from build123d import *

# Parameters (mm, degrees)
SKETCH1_R           = 3.7592
SKETCH1_R_2         = 0.6096
BOSS_EXTRUDE1_DEPTH = 1.5875
FILLET1_R           = 1.905
FILLET2_R           = 1.905


with BuildPart() as part:
    # Sketch1 → Boss-Extrude1 (new body)
    with BuildSketch(Plane.XY):
        with BuildLine():
            Line((34.29, -22.225), (33.367605666, -11.9888))
            ThreePointArc((33.367605666, -11.9888), (32.635899737, 4.284200971), (30.44668746, 20.425864572))
            ThreePointArc((30.44668746, 20.425864572), (27.794074787, 25.778474462), (22.225, 27.94))
            Line((22.225, 27.94), (-22.225, 27.94))
            ThreePointArc((-22.225, 27.94), (-27.794074787, 25.778474462), (-30.44668746, 20.425864572))
            ThreePointArc((-30.44668746, 20.425864572), (-32.635899737, 4.284200971), (-33.367605666, -11.9888))
            Line((-33.367605666, -11.9888), (-34.29, -22.225))
            Line((-34.29, -22.225), (-19.719346062, -22.225))
            ThreePointArc((-19.719346062, -22.225), (-19.755004666, -21.229024189), (-18.886028855, -21.717))
            ThreePointArc((-18.886028855, -21.717), (-18.969553044, -22.014475811), (-19.195711648, -22.225))
            Line((-19.195711648, -22.225), (19.195711648, -22.225))
            ThreePointArc((19.195711648, -22.225), (19.160053044, -21.229024189), (20.029028855, -21.717))
            ThreePointArc((20.029028855, -21.717), (19.945504666, -22.014475811), (19.719346062, -22.225))
            Line((19.719346062, -22.225), (34.29, -22.225))
        make_face()
        Polygon((-5.1562, -19.939), (-30.110080889, -19.939), (-30.110080889, -17.78), (-31.888080889, -17.78), (-31.888080889, -16.002), (-30.110080889, -16.002), (-30.110080889, -10.033), (-5.1562, -10.033), (-5.1562, -16.002), (-4.456080889, -16.002), (-4.456080889, -17.78), (-5.1562, -17.78), align=None, mode=Mode.SUBTRACT)
        with Locations((0, -15.748)):
            Circle(SKETCH1_R, mode=Mode.SUBTRACT)
        Polygon((5.1562, -19.939), (5.1562, -17.78), (4.456080889, -17.78), (4.456080889, -16.002), (5.1562, -16.002), (5.1562, -10.033), (30.110080889, -10.033), (30.110080889, -16.002), (31.888080889, -16.002), (31.888080889, -17.78), (30.110080889, -17.78), (30.110080889, -19.939), align=None, mode=Mode.SUBTRACT)
        with BuildLine():
            Line((-16.907947674, 25.654), (16.907947674, 25.654))
            ThreePointArc((16.907947674, 25.654), (17.978031977, 25.210756569), (18.421275408, 24.140672267))
            Line((18.421275408, 24.140672267), (18.421275408, 24.136275408))
            ThreePointArc((18.421275408, 24.136275408), (18.793249795, 23.238249795), (19.691275408, 22.866275408))
            Line((19.691275408, 22.866275408), (20.186724592, 22.866275408))
            ThreePointArc((20.186724592, 22.866275408), (21.084750205, 23.238249795), (21.456724592, 24.136275408))
            Line((21.456724592, 24.136275408), (21.456724592, 24.871259676))
            ThreePointArc((21.456724592, 24.871259676), (21.686749328, 25.425496663), (22.24162483, 25.653976848))
            ThreePointArc((22.24162483, 25.653976848), (26.292824304, 24.053268127), (28.177671702, 20.126203591))
            ThreePointArc((28.177671702, 20.126203591), (29.260117929, 13.484694907), (30.092217203, 6.8072))
            Line((30.092217203, 6.8072), (27.552217203, 6.8072))
            Line((27.552217203, 6.8072), (27.552217203, 4.9022))
            Line((27.552217203, 4.9022), (29.457217203, 4.9022))
            Line((29.457217203, 4.9022), (29.457217203, 3.175))
            Line((29.457217203, 3.175), (27.552217203, 3.175))
            Line((27.552217203, 3.175), (27.552217203, 1.27))
            Line((27.552217203, 1.27), (29.457217203, 1.27))
            Line((29.457217203, 1.27), (29.457217203, -5.0038))
            Line((29.457217203, -5.0038), (27.552217203, -5.0038))
            Line((27.552217203, -5.0038), (27.552217203, -6.2738))
            Line((27.552217203, -6.2738), (29.457217203, -6.2738))
            Line((29.457217203, -6.2738), (29.457217203, -8.001))
            Line((29.457217203, -8.001), (-29.457217203, -8.001))
            Line((-29.457217203, -8.001), (-29.457217203, -6.2738))
            Line((-29.457217203, -6.2738), (-27.552217203, -6.2738))
            Line((-27.552217203, -6.2738), (-27.552217203, -5.0038))
            Line((-27.552217203, -5.0038), (-29.457217203, -5.0038))
            Line((-29.457217203, -5.0038), (-29.457217203, 1.27))
            Line((-29.457217203, 1.27), (-27.552217203, 1.27))
            Line((-27.552217203, 1.27), (-27.552217203, 3.175))
            Line((-27.552217203, 3.175), (-29.457217203, 3.175))
            Line((-29.457217203, 3.175), (-29.457217203, 4.9022))
            Line((-29.457217203, 4.9022), (-27.552217203, 4.9022))
            Line((-27.552217203, 4.9022), (-27.552217203, 6.8072))
            Line((-27.552217203, 6.8072), (-30.092217203, 6.8072))
            ThreePointArc((-30.092217203, 6.8072), (-29.260117929, 13.484694907), (-28.177671702, 20.126203591))
            ThreePointArc((-28.177671702, 20.126203591), (-26.292824304, 24.053268127), (-22.24162483, 25.653976848))
            ThreePointArc((-22.24162483, 25.653976848), (-21.686749328, 25.425496663), (-21.456724592, 24.871259676))
            Line((-21.456724592, 24.871259676), (-21.456724592, 24.136275408))
            ThreePointArc((-21.456724592, 24.136275408), (-21.084750205, 23.238249795), (-20.186724592, 22.866275408))
            Line((-20.186724592, 22.866275408), (-19.691275408, 22.866275408))
            ThreePointArc((-19.691275408, 22.866275408), (-18.793249795, 23.238249795), (-18.421275408, 24.136275408))
            Line((-18.421275408, 24.136275408), (-18.421275408, 24.140672267))
            ThreePointArc((-18.421275408, 24.140672267), (-17.978031977, 25.210756569), (-16.907947674, 25.654))
        make_face(mode=Mode.SUBTRACT)
        with Locations((-19.939, 24.384)):
            Circle(SKETCH1_R_2, mode=Mode.SUBTRACT)
        with Locations((19.939, 24.384)):
            Circle(SKETCH1_R_2, mode=Mode.SUBTRACT)
    extrude(amount=BOSS_EXTRUDE1_DEPTH)

    # Fillet1
    fillet1_edges = [part.edges().sort_by_distance(p)[0] for p in [
        (5.1562, -19.939, 0.79375),
        (30.110080889, -19.939, 0.79375),
        (30.110080889, -10.033, 0.79375),
        (5.1562, -10.033, 0.79375),
        (-5.1562, -19.939, 0.79375),
        (-5.1562, -10.033, 0.79375),
        (-30.110080889, -10.033, 0.79375),
        (-30.110080889, -19.939, 0.79375),
    ]]
    fillet(fillet1_edges, radius=FILLET1_R)

    # Fillet2
    fillet2_edges = [part.edges().sort_by_distance(p)[0] for p in [
        (-29.457217203, 1.27, 0.79375),
        (-29.457217203, -5.0038, 0.79375),
        (-30.092217203, 6.8072, 0.79375),
        (29.457217203, -5.0038, 0.79375),
        (29.457217203, 1.27, 0.79375),
        (30.092217203, 6.8072, 0.79375),
    ]]
    fillet(fillet2_edges, radius=FILLET2_R - 0.0001)  # a hair under: the kernel refuses the full size


solid = part.part
Input: part model. Units: mm. Frame: model coordinates. A direction names the side the tool comes from. Coordinates: 2 decimals unless noted, no trailing zeros. Loops run counter-clockwise (first coordinate to the right, second up) from the corner with the lowest first, then second, coordinate; pieces in that order, holes last.
Q1. Contact query for flat-ended pins moving along their axis: pin 1 (0.5 mm diameter, centred on y = -17, z = 0.5, fed in from +X); pin 2 (2 mm diameter, centred on x = -19.939, y = 24.384, fed in from -Z); pin 3 (0.8 mm diameter, centred on y = 4.5, z = 0.5, fed in from -X); pin 4 (0.8 mm diameter, centred on y = -14.5, z = 1, fed in from +X). Output: stop coordinate, or through.
Q2. Draft query along X for faces 1 (the face through (29.57, -10.61, 0.8)), 2 (the face through (33.835, -17.179, 0.783)), 3 (the face through (-27.731, 25.836, 0.783)). Return one class per face: +X half, -X half, draft (parallel to the pull), parting line (faces both ways), or undercut.
Q3. Set-up query: faces 4 (the face through (5.156, -14, 1)), 5 (the face through (-0.2, -8.2, 1.588)). Return all of +Z, -Z, +X, -X, +Y, -Y with unobstructed straight access to the full face (end or side cutting, diameter ignored); none if empty.
Q4. Material intervals for line 1 (Y direction, x = -9, z = 0.6) (3 decimals); line 2 (Y direction, x = 0, z = 1.15) (3 decimals); line 3 (X direction, y = 24.5, z = 0.2), sorted ascending.
Q5. Cut plane D-D (z = 0.9). Give the number of separate pieces and of enclosed holes in the cut face, then the cut area to 3 significant figures.
Q6. Cut plane A-A (x = 13). Output: boundary loops of the cut face in (y, z) (1 decimal).
Q7. Cut plane C-C (x = 0). Output: boundary loops of the cut face in (y, z) (1 decimal), then the cut area to 3 significant figures.
Q8. Cut plane B-B (y = 13.5). Output: boundary loops of the cut face in (x, z).
Working result:
1. pin 1: stops at x = 33.84
1. pin 2: stops at z = 0
1. pin 3: stops at x = -32.65
1. pin 4: stops at x = 33.63
2. face 1: undercut
2. face 2: +X half
2. face 3: -X half
3. face 4: +Z, -Z
3. face 5: +Z, +X, -X, +Y, -Y
4. line 1: y = -22.225 to -19.939, -10.033 to -8.001, 25.654 to 27.94
4. line 2: y = -22.225 to -19.507, -11.989 to -8.001, 25.654 to 27.94
4. line 3: x = -28.93 to -25.75, -21.46 to -20.54, -19.34 to -18.38, 18.38 to 19.34, 20.54 to 21.46, 25.75 to 28.93
5. separate pieces: 1
5. enclosed holes: 6
5. area: 770 mm2
6. outline: (-22.2, 0) - (-19.9, 0) - (-19.9, 1.6) - (-22.2, 1.6) - close; (-10, 0) - (-8, 0) - (-8, 1.6) - (-10, 1.6) - close; (25.7, 0) - (27.9, 0) - (27.9, 1.6) - (25.7, 1.6) - close
7. outline: (-22.2, 0) - (-19.5, 0) - (-19.5, 1.6) - (-22.2, 1.6) - close; (-12, 0) - (-8, 0) - (-8, 1.6) - (-12, 1.6) - close; (25.7, 0) - (27.9, 0) - (27.9, 1.6) - (25.7, 1.6) - close
7. area: 14.3 mm2
8. outline: (-31.57, 0) - (-29.26, 0) - (-29.26, 1.59) - (-31.57, 1.59) - close; (29.26, 0) - (31.57, 0) - (31.57, 1.59) - (29.26, 1.59) - close
